from build123d import *

# Parameters (mm, degrees)
SKIZZE3_R                       = 1.05
SCHNITT_LINEAR_AUSTRAGEN1_DEPTH = 16.779733838
SKIZZE4_R                       = 1.9
SCHNITT_LINEAR_AUSTRAGEN2_DEPTH = 2.3
FASE1_SIZE                      = 0.1
KREISMUSTER1_COUNT              = 4
FASE1_OF_KREISMUSTER1_SIZE      = 0.1
VERRUNDUNG1_R                   = 0.1
FASE2_SIZE                      = 0.6
SKIZZE5_R                       = 1
SCHNITT_LINEAR_AUSTRAGEN3_DEPTH = 4.5
FASE3_SIZE                      = 0.2


with BuildPart() as part:
    # Skizze2 → Rotation1 (revolve)
    with BuildSketch(Plane.XY):
        Polygon((0, 0), (8, 0), (8, 3.5), (2, 3.5), (2, 14.5), (0, 14.5), align=None)
    revolve(axis=Axis((0, 0, 0), (0, 1, 0)))

    # Skizze3 → Schnitt-Linear austragen1 (cut, through all)
    with BuildSketch(Plane(origin=(0, 3.5, 0), x_dir=(1, 0, 0), z_dir=(0, 1, 0))):
        with Locations(Location((0, 4.5, 0), (0, 0, 180))):
            Circle(SKIZZE3_R)
    schnitt_linear_austragen1 = extrude(amount=-SCHNITT_LINEAR_AUSTRAGEN1_DEPTH, mode=Mode.SUBTRACT)

    # Skizze4 → Schnitt-Linear austragen2 (cut)
    with BuildSketch(Plane(origin=(0, 3.5, 0), x_dir=(1, 0, 0), z_dir=(0, 1, 0))):
        with Locations(Location((0, 4.5, 0), (0, 0, 180))):
            Circle(SKIZZE4_R)
    schnitt_linear_austragen2 = extrude(amount=-SCHNITT_LINEAR_AUSTRAGEN2_DEPTH, mode=Mode.SUBTRACT)

    # Fase1
    fase1_edges = [part.edges().sort_by_distance(p)[0] for p in [
        (1.05, 0, -4.5),
        (1.9, 3.5, -4.5),
    ]]
    chamfer(fase1_edges, length=FASE1_SIZE)

    # Kreismuster1: Schnitt-Linear austragen1, Schnitt-Linear austragen2 ×4 about axis
    kreismuster1_axis = Axis((0, 0, 0), (0, 1, 0))
    add([schnitt_linear_austragen1.rotate(kreismuster1_axis, i * 360 / KREISMUSTER1_COUNT) for i in range(1, KREISMUSTER1_COUNT)], mode=Mode.SUBTRACT)
    add([schnitt_linear_austragen2.rotate(kreismuster1_axis, i * 360 / KREISMUSTER1_COUNT) for i in range(1, KREISMUSTER1_COUNT)], mode=Mode.SUBTRACT)

    # Fase1 of Kreismuster1
    fase1_of_kreismuster1_edges = [part.edges().sort_by_distance(p)[0] for p in [
        (-4.5, 0, -1.05),
        (-4.5, 3.5, -1.9),
        (-1.05, 0, 4.5),
        (-1.9, 3.5, 4.5),
        (4.5, 0, 1.05),
        (4.5, 3.5, 1.9),
    ]]
    chamfer(fase1_of_kreismuster1_edges, length=FASE1_OF_KREISMUSTER1_SIZE)

    # Verrundung1
    verrundung1_edges = [part.edges().sort_by_distance(p)[0] for p in [
        (-2, 3.5, 0),
    ]]
    fillet(verrundung1_edges, radius=VERRUNDUNG1_R)

    # Fase2
    fase2_edges = [part.edges().sort_by_distance(p)[0] for p in [
        (-2, 14.5, 0),
    ]]
    chamfer(fase2_edges, length=FASE2_SIZE)

    # Skizze5 → Schnitt-Linear austragen3 (cut)
    with BuildSketch(Plane.XZ):
        Circle(SKIZZE5_R)
    extrude(amount=-SCHNITT_LINEAR_AUSTRAGEN3_DEPTH, mode=Mode.SUBTRACT)

    # Fase3
    fase3_edges = [part.edges().sort_by_distance(p)[0] for p in [
        (-8, 3.5, 0),
        (-8, 0, 0),
        (-1, 0, 0),
    ]]
    chamfer(fase3_edges, length=FASE3_SIZE)


solid = part.part
The listing builds one solid part. Answer for the finished solid, in the listing's coordinates (mm). A direction names the side the tool comes from. Coordinates: 2 decimals unless noted, no trailing zeros. Loops run counter-clockwise (first coordinate to the right, second up) from the corner with the lowest first, then second, coordinate; pieces in that order, holes last. Notation, with made-up numbers: (-31.5, -15.5) -> (-9.5, -15.5) arc R36 ccw to (-9.5, 19.5) -> close; hole circle Ø5 at (-22, 43). An arc over 180 degrees is marked (long way). Write item = value, one per line. Start each with the question number.
1) The mould has two halves that part along Z. Classify faces 4 (the face through (-0.247, 2.315, 2.616)), 5 (the face through (0, 14.5, 0)), 6 (the face through (0, 9, 2)): released by +Z, released by -Z, zero draft, split by the parting line, or undercut.
2) Straight lines are drawn through the part: line 1 (Z direction, x = 0, y = 0.6); line 2 (Z direction, x = 0, y = 2.15); line 3 (Y direction, x = -3.25, z = 6). For each, find the intervals that lie inside material, in ascending order. Write a range as from..to.
3) A tool of negligible diameter and unlimited length cuts with its end or side. For faces 1 (the face through (-2.616, 2.315, -0.247)), 2 (the face through (3.46, 0.66, 0.14)), 3 (the face through (0, 2, -1)), from which of +Z, -Z, +X, -X, +Y, -Y can it reach the whole face along a straight path? Write none if from no direction.
4) A cutting plane is placed at B-B (y = 10). Give the vertices of the cut face in (x, z).
5) Given pin 1 Ø1.1 at (x, z) = (0, -5.5) entering from +Y; pin 2 Ø3 at (x, y) = (1, 12) entering from +Z; pin 3 Ø1.6 at (x, z) = (0, 0) entering from -Y, each flat-ended and moving along its own axis, determine where each tip first touches the part or whether it passes through.
6) A cutting plane is placed at A-A (y = 2.25). Give the vertices of the cut face in (x, z).
Responses:
q1.face_4 = undercut
q1.face_5 = zero draft
q1.face_6 = split by the parting line
q2.line_1 = -8..-5.55, -3.45..-1, 1..3.45, 5.55..8
q2.line_2 = -8..-6.4, -2.6..-1, 1..2.6, 6.4..8
q2.line_3 = 0..3.5
q3.face_1 = +Y
q3.face_2 = +Y, -Y
q3.face_3 = -Y
q4.outline = circle Ø4 at (0, 0)
q5.pin_1 = 1.2
q5.pin_2 = 2
q5.pin_3 = 4.5
q6.outline = circle Ø16 at (0, 0); hole circle Ø3.8 at (-4.5, 0); hole circle Ø3.8 at (0, -4.5); hole circle Ø3.8 at (0, 4.5); hole circle Ø2 at (0, 0); hole circle Ø3.8 at (4.5, 0)
